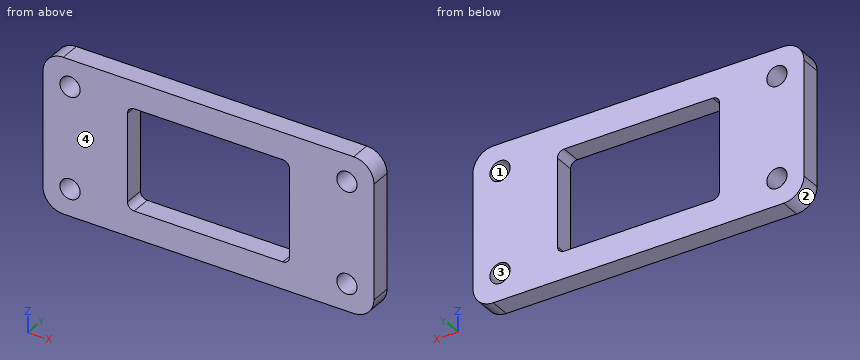
from build123d import *

# Parameters (mm, degrees)
SKETCH1_R           = 1.5
BOSS_EXTRUDE1_DEPTH = 3


with BuildPart() as part:
    # Sketch1 → Boss-Extrude1 (new body)
    with BuildSketch(Plane(origin=(0, 0, 0), x_dir=(1, 0, 0), z_dir=(0, 1, 0))):
        with BuildLine():
            Line((-4, 1), (-4, -16))
            ThreePointArc((-4, -16), (-3.121320344, -18.121320344), (-1, -19))
            Line((-1, -19), (42, -19))
            ThreePointArc((42, -19), (44.121320344, -18.121320344), (45, -16))
            Line((45, -16), (45, 1))
            ThreePointArc((45, 1), (44.121320344, 3.121320344), (42, 4))
            Line((42, 4), (-1, 4))
            ThreePointArc((-1, 4), (-3.121320344, 3.121320344), (-4, 1))
        make_face()
        Circle(SKETCH1_R, mode=Mode.SUBTRACT)
        with Locations((41, 0)):
            Circle(SKETCH1_R, mode=Mode.SUBTRACT)
        with Locations((41, -15)):
            Circle(SKETCH1_R, mode=Mode.SUBTRACT)
        with Locations((0, -15)):
            Circle(SKETCH1_R, mode=Mode.SUBTRACT)
        with BuildLine():
            Line((9.5, 0), (31.5, 0))
            ThreePointArc((31.5, 0), (32.207106781, -0.292893219), (32.5, -1))
            Line((32.5, -1), (32.5, -14))
            ThreePointArc((32.5, -14), (32.207106781, -14.707106781), (31.5, -15))
            Line((31.5, -15), (15.880823308, -15))
            Line((15.880823308, -15), (9.5, -15))
            ThreePointArc((9.5, -15), (8.792893219, -14.707106781), (8.5, -14))
            Line((8.5, -14), (8.5, -1))
            ThreePointArc((8.5, -1), (8.792893219, -0.292893219), (9.5, 0))
        make_face(mode=Mode.SUBTRACT)
    extrude(amount=BOSS_EXTRUDE1_DEPTH)


solid = part.part
The model under review builds one solid part; all positions refer to its coordinate system, in mm. Face numbers are marked on the shaded views. Round coordinates to 2 decimals unless told otherwise and drop trailing zeros. Order: outer loops, then holes, each group sorted by start corner. A loop starts at its lowest first (then second) coordinate and runs counter-clockwise, first axis right, second up. Notation, with made-up numbers: (22, 39.25) -> (51, 39.25) arc R14 ccw to (51, 64.25) -> close; hole circle Ø6 at (79.5, -11.5). An arc over 180 degrees is marked (long way). Write item = value, one per line. Start each with the question number.
Item 1: Consider section A-A on x = 41. Write out the cut boundary in (y, z), plus the area to 3 significant figures.
Item 2: Consider section C-C on x = 16.5. Write out the cut boundary in (y, z), plus the area to 3 significant figures.
Item 3: For line 1 along Z through (x, y) = (0, 1.65); line 2 along X through (y, z) = (0.7, 1); line 3 along X through (y, z) = (1.45, -0.25), list the stretches that pass through material, from the lowest coordinate up.
Item 4: Consider section D-D on y = 1.65. Write out the cut boundary in (x, z), plus the area to 3 significant figures.
Item 5: Consider section B-B on z = 10.25. Write out the cut boundary in (x, y).
Item 6: Mouldability with a two-part tool opening along Z and no side actions: class the marked faces 1, 2, 3 and 4 as released by +Z, released by -Z, zero draft, split by the parting line, or undercut.
Conclusion:
q1.outline = (0, -4) -> (3, -4) -> (3, -1.5) -> (0, -1.5) -> close; (0, 1.5) -> (3, 1.5) -> (3, 13.5) -> (0, 13.5) -> close; (0, 16.5) -> (3, 16.5) -> (3, 19) -> (0, 19) -> close
q1.area = 51.0 mm2
q2.outline = (0, -4) -> (3, -4) -> (3, 0) -> (0, 0) -> close; (0, 15) -> (3, 15) -> (3, 19) -> (0, 19) -> close
q2.area = 24.0 mm2
q3.line_1 = -4 to -1.5, 1.5 to 13.5, 16.5 to 19
q3.line_2 = -4 to -1.12, 1.12 to 8.5, 32.5 to 39.88, 42.12 to 45
q3.line_3 = -4 to -1.48, 1.48 to 39.52, 42.48 to 45
q4.outline = (-4, -1) arc R3 ccw to (-1, -4) -> (42, -4) arc R3 ccw to (45, -1) -> (45, 16) arc R3 ccw to (42, 19) -> (-1, 19) arc R3 ccw to (-4, 16) -> close; hole circle Ø3 at (0, 0); hole circle Ø3 at (0, 15); hole (8.5, 1) arc R1 ccw to (9.5, 0) -> (31.5, 0) arc R1 ccw to (32.5, 1) -> (32.5, 14) arc R1 ccw to (31.5, 15) -> (9.5, 15) arc R1 ccw to (8.5, 14) -> close; hole circle Ø3 at (41, 0); hole circle Ø3 at (41, 15)
q4.area = 732 mm2
q5.outline = (-4, 0) -> (8.5, 0) -> (8.5, 3) -> (-4, 3) -> close; (32.5, 0) -> (45, 0) -> (45, 3) -> (32.5, 3) -> close
q6.face_1 = undercut
q6.face_2 = released by -Z
q6.face_3 = undercut
q6.face_4 = zero draft
